Geometry: see drawing. Coordinates: mm, zero at the bounding-box minimum. Round coordinates to 2 decimals unless told otherwise and drop trailing zeros. Write each loop counter-clockwise with the first axis right and the second up, starting at its lowest first coordinate (ties: lowest second). Pieces come first, ordered by that corner, then holes. Notation, with made-up numbers: (77.5, -38.75) -> (94.5, -38.75) arc R20 ccw to (94.5, -32.75) -> close; hole circle Ø11 at (21, 35). An arc over 180 degrees is marked (long way). Use CSV: the item, a comma, the result in double quotes.
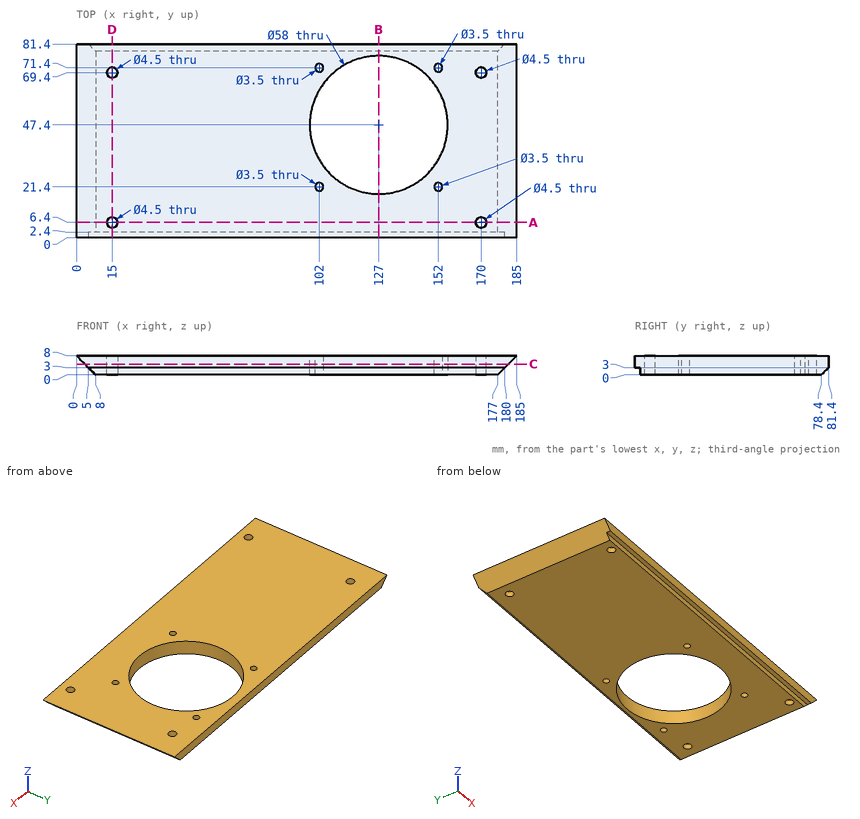
Item 1: Line query: line 1 (Y direction, x = 15, z = 4.1); line 2 (X direction, y = 69.4, z = 0.9); line 3 (X direction, y = 6, z = 4). Output: solid intervals per line, ascending.
Worked answers:
line 1,"y = 0 to 4.15, 8.65 to 67.15, 71.65 to 81.4"
line 2,"x = 7.1 to 12.75, 17.25 to 108.11, 145.89 to 167.75, 172.25 to 177.9"
line 3,"x = 4 to 12.79, 17.21 to 167.79, 172.21 to 181"
Item 2: Section query B-B on x = 127. Return the cut outline in (y, z), plus the area to 4 significant figures.
Worked answers:
outline,"(0, 3) -> (2.4, 3) -> (2.4, 0) -> (18.4, 0) -> (18.4, 8) -> (0, 8) -> close; (76.4, 0) -> (78.4, 0) -> (81.4, 3) -> (81.4, 8) -> (76.4, 8) -> close"
area,"175.5 mm²"
Item 3: Section query D-D on x = 15. Return the cut outline in (y, z).
Worked answers:
outline,"(0, 3) -> (2.4, 3) -> (2.4, 0) -> (4.15, 0) -> (4.15, 8) -> (0, 8) -> close; (8.65, 0) -> (67.15, 0) -> (67.15, 8) -> (8.65, 8) -> close; (71.65, 0) -> (78.4, 0) -> (81.4, 3) -> (81.4, 8) -> (71.65, 8) -> close"
Item 4: Section query C-C on z = 4.5. Give the number of separate pieces and of enclosed holes in the cut face, plus the area to 3 significant figures.
Worked answers:
separate pieces,"1"
enclosed holes,"9"
area,"11,700 mm²"
Item 5: First-contact query: pin 1 Ø0.9 at (x, z) = (125, 1.5) entering from -Y; pin 2 Ø2 at (y, z) = (46.5, 5) entering from -X. Flat tips, straight axial feed; report the tip coordinate or a pass-through.
Worked answers:
pin 1,"stops at y = 2.4"
pin 2,"stops at x = 2"
Item 6: Section query A-A on y = 6.4. Return the cut outline in (x, z).
Worked answers:
outline,"(0, 8) -> (8, 0) -> (12.75, 0) -> (12.75, 8) -> close; (17.25, 0) -> (167.75, 0) -> (167.75, 8) -> (17.25, 8) -> close; (172.25, 0) -> (177, 0) -> (185, 8) -> (172.25, 8) -> close"
